```python
from build123d import *

# Parameters (mm, degrees)
SKETCH1_W           = 47
SKETCH1_H           = 23
SKETCH1_W_2         = 44
SKETCH1_H_2         = 20
BOSS_EXTRUDE1_DEPTH = 13
SKETCH2_W           = 44
SKETCH2_H           = 20
CUT_EXTRUDE1_DEPTH  = 11.5
SKETCH3_W           = 8
SKETCH3_H           = 5
CUT_EXTRUDE2_DEPTH  = 11.5
CUT_EXTRUDE3_DEPTH  = 11.5
CHAMFER1_SIZE       = 0.5


with BuildPart() as part:
    # Sketch1 → Boss-Extrude1 (new body)
    with BuildSketch(Plane(origin=(0, 0, 0), x_dir=(1, 0, 0), z_dir=(0, 1, 0))):
        with Locations((0.5, -3.291122715)):
            Rectangle(SKETCH1_W, SKETCH1_H)
        with Locations((0.5, -3.291122715)):
            Rectangle(SKETCH1_W_2, SKETCH1_H_2, mode=Mode.SUBTRACT)
        with Locations((0.5, -3.291122715)):
            Rectangle(SKETCH1_W_2, SKETCH1_H_2)
    extrude(amount=BOSS_EXTRUDE1_DEPTH)

    # Sketch2 → Cut-Extrude1 (cut)
    with BuildSketch(Plane(origin=(0, 13, 0), x_dir=(1, 0, 0), z_dir=(0, 1, 0))):
        with Locations((0.5, -3.291122715)):
            Rectangle(SKETCH2_W, SKETCH2_H)
    extrude(amount=-CUT_EXTRUDE1_DEPTH, mode=Mode.SUBTRACT)

    # Sketch3 → Cut-Extrude2 (cut)
    with BuildSketch(Plane(origin=(-21.5, 0, 0), x_dir=(0, 0, -1), z_dir=(1, 0, 0))):
        with Locations((-3.291122715, 5.5)):
            Rectangle(SKETCH3_W, SKETCH3_H)
    extrude(amount=-CUT_EXTRUDE2_DEPTH, mode=Mode.SUBTRACT)

    # Sketch4 → Cut-Extrude3 (cut)
    with BuildSketch(Plane.ZY.offset(-22.5)):
        with BuildLine():
            ThreePointArc((5.291122715, 9), (3.291122715, 11), (1.291122715, 9))
            Line((1.291122715, 9), (5.291122715, 9))
        make_face()
        with BuildLine():
            Line((5.291122715, 9), (1.291122715, 9))
            ThreePointArc((1.291122715, 9), (3.291122715, 7), (5.291122715, 9))
        make_face()
        with BuildLine():
            Line((5.291122715, 13), (1.291122715, 13))
            Line((1.291122715, 13), (1.291122715, 9))
            ThreePointArc((1.291122715, 9), (3.291122715, 11), (5.291122715, 9))
            Line((5.291122715, 9), (5.291122715, 13))
        make_face()
    extrude(amount=-CUT_EXTRUDE3_DEPTH, mode=Mode.SUBTRACT)

    # Chamfer1
    chamfer1_edges = [part.edges().sort_by_distance(p)[0] for p in [
        (0.5, 0, 14.791122715),
        (-23, 0, 3.291122715),
        (0.5, 0, -8.208877285),
        (24, 0, 3.291122715),
        (24, 6.5, 14.791122715),
        (-23, 6.5, 14.791122715),
        (-23, 6.5, -8.208877285),
        (24, 6.5, -8.208877285),
    ]]
    chamfer(chamfer1_edges, length=CHAMFER1_SIZE)


solid = part.part
```
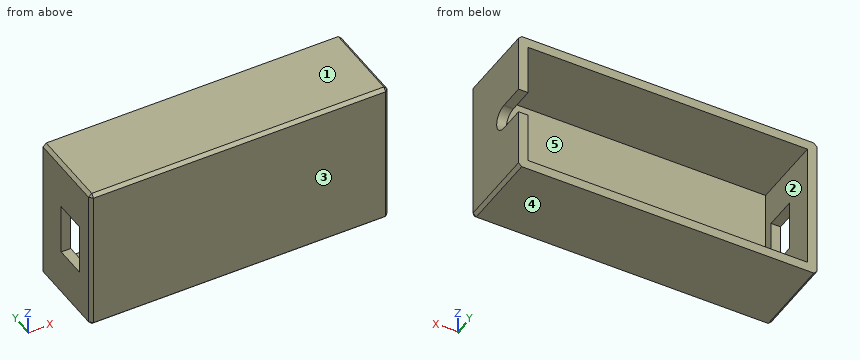
Read the model definition and answer for the solid it produces. Units are mm, in the model's axes. Face numbers are marked on the shaded views. A direction names the side the tool comes from. Coordinates: 2 decimals unless noted, no trailing zeros. Write each loop counter-clockwise with the first axis right and the second up, starting at its lowest first coordinate (ties: lowest second). Pieces come first, ordered by that corner, then holes. Notation, with made-up numbers: (21, -6) -> (58, -6) arc R7 ccw to (58, 7) -> close; hole circle Ø8 at (29.25, -7). An arc over 180 degrees is marked (long way). Answer as a JSON object with one key per item and string values.
Q1. Determine the mould class of the marked faces 3, 4 and 5 for opening direction Z: pulls with the +Z half, pulls with the -Z half, needs draft (parallel to the pull), parting line crosses it, or undercut.
The answers:
{"face 3": "needs draft", "face 4": "pulls with the -Z half", "face 5": "undercut"}
Q2. The part is cut by section D-D on x = 18.5. Give the vertices of the cut face in (y, z), then the cut area to 4 significant figures.
The answers:
{"outline": "(0, -7.71) -> (0.5, -8.21) -> (13, -8.21) -> (13, -6.71) -> (1.5, -6.71) -> (1.5, 13.29) -> (13, 13.29) -> (13, 14.79) -> (0.5, 14.79) -> (0, 14.29) -> close", "area": "68.75 mm2"}
Q3. A flat-ended cylindrical pin translates along its axis: pin 1 Ø10 at (x, z) = (-12.5, -5) entering from +Y. Find the tip coordinate at first contact, or state that the pin passes through.
The answers:
{"pin 1": "stops at y = 13"}
Q4. A tool of negligible diameter and unlimited length cuts with its end or side. For the marked faces 1 and 2, from which of +Z, -Z, +X, -X, +Y, -Y can it reach the whole face along a straight path? Write none if from no direction.
The answers:
{"face 1": "+Z, +X, -X, +Y, -Y", "face 2": "+Y"}
Q5. The part is cut by section B-B on z = 0.25. Give the vertices of the cut face in (x, y).
The answers:
{"outline": "(-23, 0.5) -> (-22.5, 0) -> (23.5, 0) -> (24, 0.5) -> (24, 13) -> (22.5, 13) -> (22.5, 1.5) -> (-21.5, 1.5) -> (-21.5, 3) -> (-23, 3) -> close; (-23, 8) -> (-21.5, 8) -> (-21.5, 13) -> (-23, 13) -> close"}
Q6. The part is cut by section C-C on y = 12.25. Give the vertices of the cut face in (x, z), then the cut area to 4 significant figures.
The answers:
{"outline": "(-23, -7.71) -> (-22.5, -8.21) -> (23.5, -8.21) -> (24, -7.71) -> (24, 1.29) -> (22.5, 1.29) -> (22.5, -6.71) -> (-21.5, -6.71) -> (-21.5, 13.29) -> (22.5, 13.29) -> (22.5, 5.29) -> (24, 5.29) -> (24, 14.29) -> (23.5, 14.79) -> (-22.5, 14.79) -> (-23, 14.29) -> close", "area": "194.5 mm2"}
Q7. The part is cut by section A-A on y = 2.5. Give the vertices of the cut face in (x, z).
The answers:
{"outline": "(-23, -7.71) -> (-22.5, -8.21) -> (23.5, -8.21) -> (24, -7.71) -> (24, 14.29) -> (23.5, 14.79) -> (-22.5, 14.79) -> (-23, 14.29) -> close; hole (-21.5, -6.71) -> (22.5, -6.71) -> (22.5, 13.29) -> (-21.5, 13.29) -> close"}
Q8. Consider line 1 (Z direction, x = 18, y = 8.25); line 2 (X direction, y = 7.5, z = 8.5); line 3 (Y direction, x = 14, z = 4.75). Determine where each line is inside the solid, lowest interval first. Write a range as [from, to].
The answers:
{"line 1": "z = [-8.21, -6.71], [13.29, 14.79]", "line 2": "x = [-23, -21.5], [22.5, 24]", "line 3": "y = [0, 1.5]"}
